```python
from build123d import *

# Parameters (mm, degrees)
SKETCH1_W           = 103
SKETCH1_H           = 30
SKETCH1_R           = 2
SKETCH1_W_2         = 7
SKETCH1_H_2         = 2
SKETCH1_W_3         = 2
SKETCH1_H_3         = 7
BOSS_EXTRUDE1_DEPTH = 2


with BuildPart() as part:
    # Sketch1 → Boss-Extrude1 (new body)
    with BuildSketch(Plane(origin=(0, 0, 0), x_dir=(1, 0, 0), z_dir=(0, 1, 0))):
        with Locations((-11.269774173, -8.963557039)):
            Rectangle(SKETCH1_W, SKETCH1_H)
        with Locations(Location((-52.769774173, -8.963557039, 0), (0, 0, 270))):
            Circle(SKETCH1_R, mode=Mode.SUBTRACT)
        with Locations(Location((30.230225827, -8.963557039, 0), (0, 0, 270))):
            Circle(SKETCH1_R, mode=Mode.SUBTRACT)
        with Locations(Location((-11.269774173, -8.963557039, 0), (0, 0, 270))):
            Circle(SKETCH1_R, mode=Mode.SUBTRACT)
        with Locations((-39.269774173, -15.463557039)):
            Rectangle(SKETCH1_W_2, SKETCH1_H_2, mode=Mode.SUBTRACT)
        with Locations((-39.269774173, -2.463557039)):
            Rectangle(SKETCH1_W_2, SKETCH1_H_2, mode=Mode.SUBTRACT)
        with Locations((16.730225827, -2.463557039)):
            Rectangle(SKETCH1_W_2, SKETCH1_H_2, mode=Mode.SUBTRACT)
        with Locations((16.730225827, -15.463557039)):
            Rectangle(SKETCH1_W_2, SKETCH1_H_2, mode=Mode.SUBTRACT)
        with Locations((-29.769774173, -2.463557039)):
            Rectangle(SKETCH1_W_3, SKETCH1_H_3, mode=Mode.SUBTRACT)
        with Locations((-29.769774173, -15.463557039)):
            Rectangle(SKETCH1_W_3, SKETCH1_H_3, mode=Mode.SUBTRACT)
        with Locations((7.230225827, -15.463557039)):
            Rectangle(SKETCH1_W_3, SKETCH1_H_3, mode=Mode.SUBTRACT)
        with Locations((7.230225827, -2.463557039)):
            Rectangle(SKETCH1_W_3, SKETCH1_H_3, mode=Mode.SUBTRACT)
    extrude(amount=BOSS_EXTRUDE1_DEPTH)


solid = part.part
```
Read the model definition and answer for the solid it produces. Units are mm, in the model's axes. A direction names the side the tool comes from. Give positions to 0.01 mm unless a question says otherwise; leave off trailing zeros. Write each loop counter-clockwise with the first axis right and the second up, starting at its lowest first coordinate (ties: lowest second). Pieces come first, ordered by that corner, then holes. Notation, with made-up numbers: (35, 31) - (50, 31) arc R9 cw to (50, 45) - close; hole circle Ø1 at (-30, 65). An arc over 180 degrees is marked (long way). Write item = value, one per line. Start each with the question number.
Item 1: Each of these flat-tipped pins is pushed along its axis until it touches: P1, Ø6, axis at x = -7, z = 20.5, coming from the -Y side; P2, Ø3.5, axis at x = -52.77, z = 8.96, coming from the -Y side. Where does it stop, or does it pass through?
Item 2: Find section C-C (y = 0.4). State how many separate pieces and enclosed holes the cut face has, then the cut area to 3 significant figures.
Item 3: Find the intervals of material crossed by probe 1 along X at (y, z) = (1.35, 16.25); probe 2 along X at (y, z) = (1.85, 17.25); probe 3 along Z at (x, y) = (18, 1.05), in increasing order. Write a range as [from, to].
Item 4: Find section A-A (z = 5). Give the vertices of the cut face in (x, y).
Item 5: Find section B-B (x = -38). Give the vertices of the cut face in (y, z), then the cut area to 3 significant figures.
Item 6: A tool of negligible diameter and unlimited length cuts with its end or side. For faces 4 (the flat face through (-42.77, 1, 15)), 5 (the flat face through (-12, 0, 12)), from which of +Z, -Z, +X, -X, +Y, -Y can it reach the whole face along a straight path? Write none if from no direction.
Item 7: The mould has two halves that part along X. Classify faces 1 (the flat face through (-12, 1, 23.964)), 2 (the flat face through (40.23, 1, 9)), 3 (the cylindrical face through (-50.787, 0.986, 8.703)): +X half, -X half, draft (parallel to the pull), parting line (faces both ways), or undercut.
Response:
q1.P1 = 0
q1.P2 = through
q2.separate_pieces = 1
q2.enclosed_holes = 11
q2.area = 2,940 mm²
q3.probe_1 = [-62.77, -42.77], [-35.77, -30.77], [-28.77, 6.23], [8.23, 13.23], [20.23, 40.23]
q3.probe_2 = [-62.77, -30.77], [-28.77, 6.23], [8.23, 40.23]
q3.probe_3 = [-6.04, 1.46], [3.46, 14.46], [16.46, 23.96]
q4.outline = (-62.77, 0) - (-30.77, 0) - (-30.77, 2) - (-62.77, 2) - close; (-28.77, 0) - (6.23, 0) - (6.23, 2) - (-28.77, 2) - close; (8.23, 0) - (40.23, 0) - (40.23, 2) - (8.23, 2) - close
q5.outline = (0, -6.04) - (2, -6.04) - (2, 1.46) - (0, 1.46) - close; (0, 3.46) - (2, 3.46) - (2, 14.46) - (0, 14.46) - close; (0, 16.46) - (2, 16.46) - (2, 23.96) - (0, 23.96) - close
q5.area = 52.0 mm²
q6.face_4 = +Y, -Y
q6.face_5 = +Z, -Z, +X, -X, -Y
q7.face_1 = draft
q7.face_2 = +X half
q7.face_3 = undercut
